from build123d import *

# Parameters (mm, degrees)
SKETCH1_R           = 18.5
BOSS_EXTRUDE1_DEPTH = 23.016176471
SKETCH2_R           = 18.1
BOSS_EXTRUDE2_DEPTH = 33.3
SKETCH3_R           = 6
BOSS_EXTRUDE3_DEPTH = 5
BOSS_EXTRUDE4_DEPTH = 15
CUT_EXTRUDE1_START  = -14
CUT_EXTRUDE1_DEPTH  = 14
SKETCH6_R           = 1.5
CUT_EXTRUDE2_DEPTH  = 8


with BuildPart() as part:
    # Sketch1 → Boss-Extrude1 (new body)
    with BuildSketch(Plane.XY):
        Circle(SKETCH1_R)
    extrude(amount=BOSS_EXTRUDE1_DEPTH)

    # Sketch2 → Boss-Extrude2 (add)
    with BuildSketch(Plane.XY.offset(23.016176471)):
        Circle(SKETCH2_R)
    extrude(amount=BOSS_EXTRUDE2_DEPTH)

    # Sketch3 → Boss-Extrude3 (add)
    with BuildSketch(Plane(origin=(0, 0, 0), x_dir=(-1, 0, 0), z_dir=(0, 0, -1))):
        Circle(SKETCH3_R)
    extrude(amount=BOSS_EXTRUDE3_DEPTH)

    # Sketch4 → Boss-Extrude4 (add)
    with BuildSketch(Plane(origin=(0, 0, -5), x_dir=(-1, 0, 0), z_dir=(0, 0, -1))):
        with BuildLine():
            ThreePointArc((-0.515876955, 2.95531233), (0, -3), (0.515876955, 2.95531233))
            ThreePointArc((0.515876955, 2.95531233), (0, 3), (-0.515876955, 2.95531233))
        make_face()
    extrude(amount=BOSS_EXTRUDE4_DEPTH)

    # Sketch5 → Cut-Extrude1 (cut)
    with BuildSketch(Plane(origin=(0, 0, -20), x_dir=(-1, 0, 0), z_dir=(0, 0, -1)).offset(CUT_EXTRUDE1_START)):
        with BuildLine():
            Line((-1.658312395, 2.5), (1.658312395, 2.5))
            ThreePointArc((1.658312395, 2.5), (0, 3), (-1.658312395, 2.5))
        make_face()
    extrude(amount=CUT_EXTRUDE1_DEPTH, mode=Mode.SUBTRACT)

    # Sketch6 → Cut-Extrude2 (cut)
    with BuildSketch(Plane(origin=(0, 0, 0), x_dir=(-1, 0, 0), z_dir=(0, 0, -1))):
        with Locations((7.75, 13.423393759)):
            Circle(SKETCH6_R)
        with Locations((15.5, 0)):
            Circle(SKETCH6_R)
        with Locations((7.75, -13.423393759)):
            Circle(SKETCH6_R)
        with Locations((-7.75, -13.423393759)):
            Circle(SKETCH6_R)
        with Locations((-15.5, 0)):
            Circle(SKETCH6_R)
        with Locations((-7.75, 13.423393759)):
            Circle(SKETCH6_R)
    extrude(amount=-CUT_EXTRUDE2_DEPTH, mode=Mode.SUBTRACT)


solid = part.part
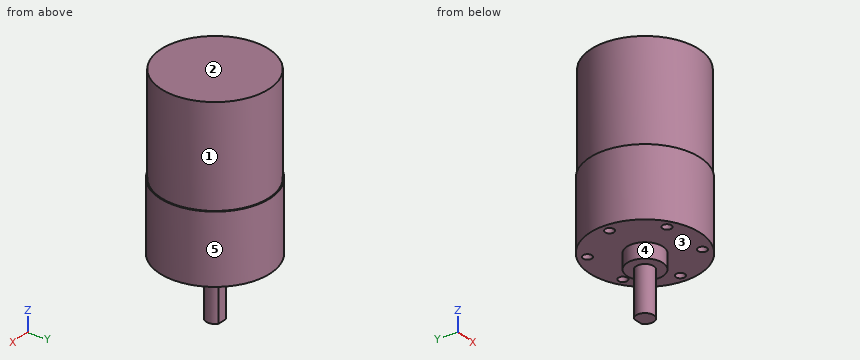
Read the model definition and answer for the solid it produces. Units are mm, in the model's axes. Face numbers are marked on the shaded views. A direction names the side the tool comes from. Give positions to 0.01 mm unless a question says otherwise; leave off trailing zeros. Write each loop counter-clockwise with the first axis right and the second up, starting at its lowest first coordinate (ties: lowest second). Pieces come first, ordered by that corner, then holes. Notation, with made-up numbers: (70.25, -39.75) - (117.25, -39.75) arc R32 ccw to (117.25, -0.75) - close; hole circle Ø2 at (36.25, 41). An arc over 180 degrees is marked (long way). Answer in a Markdown table with one row per item. Add a question column.
Item 1: Determine the mould class of the marked faces 1, 2 and 3 for opening direction Z: pulls with the +Z half, pulls with the -Z half, needs draft (parallel to the pull), parting line crosses it, or undercut.
Item 2: Section C-C, the plane x = -15.5 is taken. Write down the section's boundary in (y, z), and give its area (3 significant figures).
Item 3: Section A-A, the plane y = 0 is taken. Write down the section's boundary in (x, z), and give its area (3 significant figures).
Item 4: A tool of negligible diameter and unlimited length cuts with its end or side. For the marked faces 4 and 5, from which of +Z, -Z, +X, -X, +Y, -Y can it reach the whole face along a straight path? Write none if from no direction.
Item 5: Section B-B, the plane z = 6 is taken. Write down the section's boundary in (x, y), and give its area (3 significant figures).
Item 6: Section D-D, the plane z = -14 is taken. Write down the section's boundary in (x, y), and give its area (3 significant figures).
Item 7: Find the intervals of material crossed by L1, parallel to Y at x = 7, z = 5; L2, parallel to Z at x = -6.5, y = -8.5; L3, parallel to Y at x = -7.75, z = 6.5, in increasing order.
Item 8: Flat-ended cylindrical pins translate along their axes: P1, Ø3.5, axis at x = 7.75, y = -13.42, coming from the -Z side; P2, Ø1.5, axis at y = -3, z = 43.5, coming from the -X side; P3, Ø0.9, axis at x = 16, y = -0.5, coming from the -Z side; P4, Ø1.5, axis at x = -14, y = 13.5, coming from the -Z side. Find the tip coordinate at first contact, or state that the pin passes through.
Recorded:
| question | item | result |
|---|---|---|
| 1 | face 1 | needs draft |
| 1 | face 2 | pulls with the +Z half |
| 1 | face 3 | pulls with the -Z half |
| 2 | outline | (-10.1, 0) - (-1.5, 0) - (-1.5, 8) - (1.5, 8) - (1.5, 0) - (10.1, 0) - (10.1, 23.02) - (9.35, 23.02) - (9.35, 56.32) - (-9.35, 56.32) - (-9.35, 23.02) - (-10.1, 23.02) - close |
| 2 | area | 1,060 mm2 |
| 3 | outline | (-18.5, 0) - (-17, 0) - (-17, 8) - (-14, 8) - (-14, 0) - (-6, 0) - (-6, -5) - (-3, -5) - (-3, -20) - (3, -20) - (3, -5) - (6, -5) - (6, 0) - (14, 0) - (14, 8) - (17, 8) - (17, 0) - (18.5, 0) - (18.5, 23.02) - (18.1, 23.02) - (18.1, 56.32) - (-18.1, 56.32) - (-18.1, 23.02) - (-18.5, 23.02) - close |
| 3 | area | 2,160 mm2 |
| 4 | face 4 | -Z |
| 4 | face 5 | +Z, -Z |
| 5 | outline | circle Ø37 at (0, 0); hole circle Ø3 at (-15.5, 0); hole circle Ø3 at (-7.75, -13.42); hole circle Ø3 at (-7.75, 13.42); hole circle Ø3 at (7.75, -13.42); hole circle Ø3 at (7.75, 13.42); hole circle Ø3 at (15.5, 0) |
| 5 | area | 1,030 mm2 |
| 6 | outline | (-1.66, 2.5) arc R3 ccw (long way) to (1.66, 2.5) - close |
| 6 | area | 27.1 mm2 |
| 7 | L1 | y = -17.12 to -14.72, -12.12 to 12.12, 14.72 to 17.12 |
| 7 | L2 | z = 0 to 56.32 |
| 7 | L3 | y = -16.8 to -14.92, -11.92 to 11.92, 14.92 to 16.8 |
| 8 | P1 | stops at z = 0 |
| 8 | P2 | stops at x = -17.96 |
| 8 | P3 | stops at z = 8 |
| 8 | P4 | passes through |
